from build123d import *

# Parameters (mm, degrees)
CROQUIS1_W              = 10.45
CROQUIS1_H              = 13.3
CROQUIS1_R              = 1.4
SALIENTE_EXTRUIR1_DEPTH = 1.66
SALIENTE_EXTRUIR2_DEPTH = 1
SALIENTE_EXTRUIR3_DEPTH = 0.6
CROQUIS4_R              = 0.5
CORTAR_EXTRUIR1_DEPTH   = 2
CROQUIS5_W              = 1.18
CROQUIS5_H              = 3
SALIENTE_EXTRUIR4_DEPTH = 1
CROQUIS6_R              = 0.670494612
CROQUIS6_R_2            = 0.5
CROQUIS6_R_3            = 0.673168706
CROQUIS6_R_4            = 1.920139837
CROQUIS6_R_5            = 1.4
SALIENTE_EXTRUIR5_DEPTH = 0.1
CROQUIS7_W              = 0.8
CROQUIS7_H              = 0.488253232
CROQUIS7_W_2            = 0.85
CROQUIS7_W_3            = 0.528941002
CROQUIS7_H_2            = 0.8
CORTAR_EXTRUIR2_DEPTH   = 0.1


with BuildPart() as part:
    # Croquis1 → Saliente-Extruir1 (new body)
    with BuildSketch(Plane.XY):
        Rectangle(CROQUIS1_W, CROQUIS1_H)
        with Locations((-2.775, 3.86)):
            Circle(CROQUIS1_R, mode=Mode.SUBTRACT)
    extrude(amount=SALIENTE_EXTRUIR1_DEPTH)

    # Croquis2 → Saliente-Extruir2 (add)
    with BuildSketch(Plane.XY.offset(1.66)):
        with BuildLine():
            Line((1.014875741, 5.05), (4.064875741, 5.05))
            ThreePointArc((4.064875741, 5.05), (4.13558642, 5.020710678), (4.164875741, 4.95))
            Line((4.164875741, 4.95), (4.164875741, 1.9))
            ThreePointArc((4.164875741, 1.9), (4.13558642, 1.829289322), (4.064875741, 1.8))
            Line((4.064875741, 1.8), (1.014875741, 1.8))
            ThreePointArc((1.014875741, 1.8), (0.944165063, 1.829289322), (0.914875741, 1.9))
            Line((0.914875741, 1.9), (0.914875741, 4.95))
            ThreePointArc((0.914875741, 4.95), (0.944165063, 5.020710678), (1.014875741, 5.05))
        make_face()
    extrude(amount=SALIENTE_EXTRUIR2_DEPTH)

    # Croquis3 → Saliente-Extruir3 (add)
    with BuildSketch(Plane.XY.offset(1.66)):
        with BuildLine():
            Line((0.545086024, -4.450002724), (-0.029222615, -4.450002724))
            ThreePointArc((-0.029222615, -4.450002724), (-0.109016561, -4.41695099), (-0.142068295, -4.337157044))
            Line((-0.142068295, -4.337157044), (-0.142068295, -2.862848405))
            ThreePointArc((-0.142068295, -2.862848405), (-0.109016561, -2.783054459), (-0.029222615, -2.750002724))
            Line((-0.029222615, -2.750002724), (0.545086024, -2.750002724))
            ThreePointArc((0.545086024, -2.750002724), (0.62487997, -2.783054459), (0.657931705, -2.862848405))
            Line((0.657931705, -2.862848405), (0.657931705, -4.337157044))
            ThreePointArc((0.657931705, -4.337157044), (0.62487997, -4.41695099), (0.545086024, -4.450002724))
        make_face()
        with BuildLine():
            Line((-4.549824975, -4.337157044), (-4.549824975, -2.862848405))
            ThreePointArc((-4.549824975, -2.862848405), (-4.516773241, -2.783054459), (-4.436979295, -2.750002724))
            Line((-4.436979295, -2.750002724), (-3.862670656, -2.750002724))
            ThreePointArc((-3.862670656, -2.750002724), (-3.78287671, -2.783054459), (-3.749824975, -2.862848405))
            Line((-3.749824975, -2.862848405), (-3.749824975, -4.337157044))
            ThreePointArc((-3.749824975, -4.337157044), (-3.78287671, -4.41695099), (-3.862670656, -4.450002724))
            Line((-3.862670656, -4.450002724), (-4.436979295, -4.450002724))
            ThreePointArc((-4.436979295, -4.450002724), (-4.516773241, -4.41695099), (-4.549824975, -4.337157044))
        make_face()
        with BuildLine():
            Line((3.58895412, -2.716727386), (4.213262759, -2.716727386))
            ThreePointArc((4.213262759, -2.716727386), (4.293056705, -2.749779121), (4.32610844, -2.829573067))
            Line((4.32610844, -2.829573067), (4.32610844, -4.303881706))
            ThreePointArc((4.32610844, -4.303881706), (4.293056705, -4.383675652), (4.213262759, -4.416727386))
            Line((4.213262759, -4.416727386), (3.58895412, -4.416727386))
            ThreePointArc((3.58895412, -4.416727386), (3.509160174, -4.383675652), (3.47610844, -4.303881706))
            Line((3.47610844, -4.303881706), (3.47610844, -2.829573067))
            ThreePointArc((3.47610844, -2.829573067), (3.509160174, -2.749779121), (3.58895412, -2.716727386))
        make_face()
        with BuildLine():
            Line((1.661189231, -4.337157044), (1.661189231, -2.862848405))
            ThreePointArc((1.661189231, -2.862848405), (1.694240966, -2.783054459), (1.774034912, -2.750002724))
            Line((1.774034912, -2.750002724), (2.398343551, -2.750002724))
            ThreePointArc((2.398343551, -2.750002724), (2.478137497, -2.783054459), (2.511189231, -2.862848405))
            Line((2.511189231, -2.862848405), (2.511189231, -4.337157044))
            ThreePointArc((2.511189231, -4.337157044), (2.478137497, -4.41695099), (2.398343551, -4.450002724))
            Line((2.398343551, -4.450002724), (1.774034912, -4.450002724))
            ThreePointArc((1.774034912, -4.450002724), (1.694240966, -4.41695099), (1.661189231, -4.337157044))
        make_face()
        with BuildLine():
            Line((1.689875741, 0.350979107), (1.689875741, 0.925287746))
            ThreePointArc((1.689875741, 0.925287746), (1.722927476, 1.005081692), (1.802721422, 1.038133426))
            Line((1.802721422, 1.038133426), (3.277030061, 1.038133426))
            ThreePointArc((3.277030061, 1.038133426), (3.356824007, 1.005081692), (3.389875741, 0.925287746))
            Line((3.389875741, 0.925287746), (3.389875741, 0.350979107))
            ThreePointArc((3.389875741, 0.350979107), (3.356824007, 0.271185161), (3.277030061, 0.238133426))
            Line((3.277030061, 0.238133426), (1.802721422, 0.238133426))
            ThreePointArc((1.802721422, 0.238133426), (1.722927476, 0.271185161), (1.689875741, 0.350979107))
        make_face()
    extrude(amount=SALIENTE_EXTRUIR3_DEPTH)

    # Croquis4 → Cortar-Extruir1 (cut)
    with BuildSketch(Plane.XY.offset(1.66)):
        with Locations((4.194245203, -5.773988592)):
            Circle(CROQUIS4_R)
        with Locations((1.394245203, -5.773988592)):
            Circle(CROQUIS4_R)
        with Locations((-1.405754797, -5.773988592)):
            Circle(CROQUIS4_R)
        with Locations((-4.205754797, -5.773988592)):
            Circle(CROQUIS4_R)
    extrude(amount=-CORTAR_EXTRUIR1_DEPTH, mode=Mode.SUBTRACT)

    # Croquis5 → Saliente-Extruir4 (add)
    with BuildSketch(Plane.XY.offset(1.66)):
        with Locations((-1.72406111, -2.950002724)):
            Rectangle(CROQUIS5_W, CROQUIS5_H)
    extrude(amount=SALIENTE_EXTRUIR4_DEPTH)

    # Croquis6 → Saliente-Extruir5 (add)
    with BuildSketch(Plane.XY.offset(1.66)):
        with Locations((-4.205754797, -5.773988592)):
            Circle(CROQUIS6_R)
        with Locations((-4.205754797, -5.773988592)):
            Circle(CROQUIS6_R_2, mode=Mode.SUBTRACT)
        with Locations((-1.405754797, -5.773988592)):
            Circle(CROQUIS6_R)
        with Locations((-1.405754797, -5.773988592)):
            Circle(CROQUIS6_R_2, mode=Mode.SUBTRACT)
        with Locations((1.394245203, -5.773988592)):
            Circle(CROQUIS6_R)
        with Locations((1.394245203, -5.773988592)):
            Circle(CROQUIS6_R_2, mode=Mode.SUBTRACT)
        with Locations((4.194245203, -5.773988592)):
            Circle(CROQUIS6_R_3)
        with Locations((4.194245203, -5.773988592)):
            Circle(CROQUIS6_R_2, mode=Mode.SUBTRACT)
        with Locations((-2.775, 3.86)):
            Circle(CROQUIS6_R_4)
        with Locations((-2.775, 3.86)):
            Circle(CROQUIS6_R_5, mode=Mode.SUBTRACT)
    extrude(amount=SALIENTE_EXTRUIR5_DEPTH)

    # Croquis7 → Cortar-Extruir2 (cut)
    with BuildSketch(Plane.XY.offset(2.26)):
        with Locations((-4.149824975, -3.600867586)):
            Rectangle(CROQUIS7_W, CROQUIS7_H)
        with Locations((0.257931705, -3.600867586)):
            Rectangle(CROQUIS7_W, CROQUIS7_H)
        with Locations((2.086189231, -3.600867586)):
            Rectangle(CROQUIS7_W_2, CROQUIS7_H)
        with Locations((3.90110844, -3.600867586)):
            Rectangle(CROQUIS7_W_2, CROQUIS7_H)
        with Locations((2.563329468, 0.638133426)):
            Rectangle(CROQUIS7_W_3, CROQUIS7_H_2)
    extrude(amount=-CORTAR_EXTRUIR2_DEPTH, mode=Mode.SUBTRACT)


solid = part.part
For this review, take the finished solid that the model builds, in its own axes (mm). Round coordinates to 2 decimals unless told otherwise and drop trailing zeros. Loops run counter-clockwise (first coordinate to the right, second up) from the corner with the lowest first, then second, coordinate; pieces in that order, holes last. Notation, with made-up numbers: (38.5, -1) - (95.5, -1) arc R16 cw to (95.5, 12) - close; hole circle Ø7 at (83, 38.25). An arc over 180 degrees is marked (long way). Put each result on its own line as item: value. Start each with the question number.
1. Consider section D-D on z = 0.4. State the section outline as (x, y) points (3 decimals), plus the area to 3 significant figures.
2. Insertion check: P1, Ø0.6, axis at x = 4, y = -4.5, coming from the +Z side; P2, Ø0.6, axis at x = 0.5, z = 2, coming from the +Y side. Each pin has a flat end and moves straight along its axis. Give the tip position at first contact, or say it passes through.
3. For probe 1 along X at (y, z) = (-4, 1.9); probe 2 along Z at (x, y) = (0, -1.75); probe 3 along Y at (x, z) = (1.75, 2.2) (3 decimals), list the stretches that pass through material, from the lowest coordinate up. Write a range as [from, to].
4. Consider section B-B on x = -2.5. State the section outline as (y, z) points, plus the area to 3 significant figures.
5. Mouldability with a two-part tool opening along Y and no side actions: class faces 1 (the flat face through (3, 1.8, 2)), 2 (the flat face through (0, -6.65, 1)), 3 (the flat face through (0.915, 3, 2)) as +Y half, -Y half, draft (parallel to the pull), parting line (faces both ways), or undercut.
6. Consider section A-A on y = 3.86. State the section outline as (x, z) points (3 decimals).
7. Consider section C-C on y = -1.75. State the section outline as (x, z) points (3 decimals), plus the area to 3 significant figures.
Result sheet:
1. outline: (-5.225, -6.65) - (5.225, -6.65) - (5.225, 6.65) - (-5.225, 6.65) - close; hole circle Ø1 at (-4.206, -5.774); hole circle Ø2.8 at (-2.775, 3.86); hole circle Ø1 at (-1.406, -5.774); hole circle Ø1 at (1.394, -5.774); hole circle Ø1 at (4.194, -5.774)
1. area: 130 mm^2
2. P1: z = 2.26
2. P2: y = -2.75
3. probe 1: [-4.55, -3.75], [-2.31, -1.13], [-0.14, 0.66], [1.66, 2.51], [3.48, 4.33]
3. probe 2: [0, 1.66]
3. probe 3: [-4.447, -3.845], [-3.357, -2.753], [0.251, 1.025], [1.8, 5.05]
4. outline: (-6.65, 0) - (2.49, 0) - (2.49, 1.76) - (1.96, 1.76) - (1.96, 1.66) - (-6.65, 1.66) - close; (5.23, 0) - (6.65, 0) - (6.65, 1.66) - (5.76, 1.66) - (5.76, 1.76) - (5.23, 1.76) - close
4. area: 17.6 mm^2
5. face 1: undercut
5. face 2: -Y half
5. face 3: draft
6. outline: (-5.225, 0) - (-4.175, 0) - (-4.175, 1.76) - (-4.695, 1.76) - (-4.695, 1.66) - (-5.225, 1.66) - close; (-1.375, 0) - (5.225, 0) - (5.225, 1.66) - (4.165, 1.66) - (4.165, 2.66) - (0.915, 2.66) - (0.915, 1.66) - (-0.855, 1.66) - (-0.855, 1.76) - (-1.375, 1.76) - close
7. outline: (-5.225, 0) - (5.225, 0) - (5.225, 1.66) - (-1.134, 1.66) - (-1.134, 2.66) - (-2.314, 2.66) - (-2.314, 1.66) - (-5.225, 1.66) - close
7. area: 18.5 mm^2
